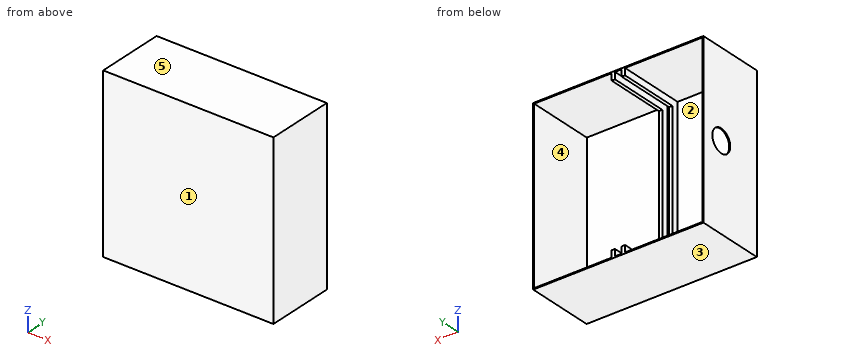
```python
from build123d import *

# Parameters (mm, degrees)
SKETCH1_W           = 253
SKETCH1_H           = 253
BOSS_EXTRUDE1_DEPTH = 101.5
SHELL2_T            = -1.5
SKETCH2_W           = 5
SKETCH2_H           = 230
BOSS_EXTRUDE3_DEPTH = 10
SKETCH3_W           = 5
SKETCH3_H           = 10
BOSS_EXTRUDE4_DEPTH = 100
SKETCH4_R           = 17
CUT_EXTRUDE1_DEPTH  = 1.5


with BuildPart() as part:
    # Sketch1 → Boss-Extrude1 (new body)
    with BuildSketch(Plane(origin=(0, 0, 0), x_dir=(1, 0, 0), z_dir=(0, 1, 0))):
        Rectangle(SKETCH1_W, SKETCH1_H)
    extrude(amount=BOSS_EXTRUDE1_DEPTH)

    # Shell2
    shell2_openings = [part.faces().sort_by_distance(p)[0] for p in [
        (0, 101.5, 0),
    ]]
    offset(amount=SHELL2_T, openings=shell2_openings, kind=Kind.INTERSECTION)

    # Sketch2 → Boss-Extrude3 (add)
    with BuildSketch(Plane(origin=(0, 1.5, 0), x_dir=(1, 0, 0), z_dir=(0, 1, 0))):
        with Locations((-7.5, 0)):
            Rectangle(SKETCH2_W, SKETCH2_H)
        with Locations((7.5, 0)):
            Rectangle(SKETCH2_W, SKETCH2_H)
    extrude(amount=BOSS_EXTRUDE3_DEPTH)

    # Sketch3 → Boss-Extrude4 (add)
    with BuildSketch(Plane(origin=(0, 1.5, 0), x_dir=(1, 0, 0), z_dir=(0, 1, 0))):
        with Locations((-7.5, 120)):
            Rectangle(SKETCH3_W, SKETCH3_H)
        with Locations((7.5, 120)):
            Rectangle(SKETCH3_W, SKETCH3_H)
        with Locations((7.5, -120)):
            Rectangle(SKETCH3_W, SKETCH3_H)
        with Locations((-7.5, -120)):
            Rectangle(SKETCH3_W, SKETCH3_H)
    extrude(amount=BOSS_EXTRUDE4_DEPTH)

    # Sketch4 → Cut-Extrude1 (cut)
    with BuildSketch(Plane.ZY.offset(126.5)):
        with Locations((0, 67.5)):
            Circle(SKETCH4_R)
    extrude(amount=-CUT_EXTRUDE1_DEPTH, mode=Mode.SUBTRACT)


solid = part.part
```
The listing builds one solid part. Answer for the finished solid, in the listing's coordinates (mm). Face numbers are marked on the shaded views. A direction names the side the tool comes from. Coordinates: 2 decimals unless noted, no trailing zeros. Write each loop counter-clockwise with the first axis right and the second up, starting at its lowest first coordinate (ties: lowest second). Pieces come first, ordered by that corner, then holes. Notation, with made-up numbers: (23, 4) - (38, 4) arc R15 cw to (38, 10) - close; hole circle Ø8 at (89.5, -27.5). An arc over 180 degrees is marked (long way). Return JSON: item names as keys, results as strings. Group by question number.
Q1. Which of the six approach directions +Z, -Z, +X, -X, +Y, -Y give full straight-line access (tool end or side, diameter ignored) to the marked faces 4 and 5?
Q2. Find the intervals of material crossed by line 1 along X through (y, z) = (8.5, 6); line 2 along X through (y, z) = (91.5, 105), in increasing order. Write a range as [from, to].
Q3. The part is cut by section B-B on y = 59.5. Write down the section's boundary in (x, z), and give its area (3 significant figures).
Q4. For a pull along Z with two mould halves and no side action, classify the marked faces 1, 2 and 3 as +Z half, -Z half, draft (parallel to the pull), parting line (faces both ways), or undercut.
Q5. The part is cut by section A-A on z = 0. Write down the section's boundary in (x, y), and give its area (4 significant figures).
Q6. Flat-ended cylindrical pins translate along their axes: pin 1 Ø1.5 at (x, z) = (-6.5, 15) entering from +Y; pin 2 Ø2 at (x, z) = (-43.5, -53.5) entering from +Y. Find the tip coordinate at first contact, or state that the pin passes through.
Q7. The part is cut by section C-C on y = 33. Write down the section's boundary in (x, z).
Q8. The part is cut by section D-D on z = 91. Write down the section's boundary in (x, y).
Evaluation:
{
 "1": {"face 4": "+Y", "face 5": "+Z, +X, -X, +Y, -Y"},
 "2": {"line 1": "x = [-126.5, -125], [-10, -5], [5, 10], [125, 126.5]", "line 2": "x = [-126.5, -125], [125, 126.5]"},
 "3": {"outline": "(-126.5, -126.5) - (126.5, -126.5) - (126.5, 126.5) - (-126.5, 126.5) - (-126.5, 15) - (-125, 15) - (-125, 125) - (-10, 125) - (-10, 115) - (-5, 115) - (-5, 125) - (5, 125) - (5, 115) - (10, 115) - (10, 125) - (125, 125) - (125, -125) - (10, -125) - (10, -115) - (5, -115) - (5, -125) - (-5, -125) - (-5, -115) - (-10, -115) - (-10, -125) - (-125, -125) - (-125, -15) - (-126.5, -15) - close", "area": "1,660 mm2"},
 "4": {"face 1": "draft", "face 2": "undercut", "face 3": "-Z half"},
 "5": {"outline": "(-126.5, 0) - (126.5, 0) - (126.5, 101.5) - (125, 101.5) - (125, 1.5) - (10, 1.5) - (10, 11.5) - (5, 11.5) - (5, 1.5) - (-5, 1.5) - (-5, 11.5) - (-10, 11.5) - (-10, 1.5) - (-125, 1.5) - (-125, 50.5) - (-126.5, 50.5) - close; (-126.5, 84.5) - (-125, 84.5) - (-125, 101.5) - (-126.5, 101.5) - close", "area": "728.5 mm2"},
 "6": {"pin 1": "stops at y = 11.5", "pin 2": "stops at y = 1.5"},
 "7": {"outline": "(-126.5, -126.5) - (126.5, -126.5) - (126.5, 126.5) - (-126.5, 126.5) - close; hole (-125, -125) - (-10, -125) - (-10, -115) - (-5, -115) - (-5, -125) - (5, -125) - (5, -115) - (10, -115) - (10, -125) - (125, -125) - (125, 125) - (10, 125) - (10, 115) - (5, 115) - (5, 125) - (-5, 125) - (-5, 115) - (-10, 115) - (-10, 125) - (-125, 125) - close"},
 "8": {"outline": "(-126.5, 0) - (126.5, 0) - (126.5, 101.5) - (125, 101.5) - (125, 1.5) - (10, 1.5) - (10, 11.5) - (5, 11.5) - (5, 1.5) - (-5, 1.5) - (-5, 11.5) - (-10, 11.5) - (-10, 1.5) - (-125, 1.5) - (-125, 101.5) - (-126.5, 101.5) - close"}
}
